from build123d import *

# Parameters (mm, degrees)
BOSS_EXTRUDE1_DEPTH = 3.175


with BuildPart() as part:
    # Sketch1 → Boss-Extrude1 (new body, symmetric)
    with BuildSketch(Plane(origin=(0, 0, 0), x_dir=(1, 0, 0), z_dir=(0, 1, 0))):
        Polygon((-203.2, 0), (203.2, 0), (203.2, 50.8), (82.55, 177.8), (-82.55, 177.8), (-203.2, 50.8), align=None)
    extrude(amount=BOSS_EXTRUDE1_DEPTH, both=True)


solid = part.part
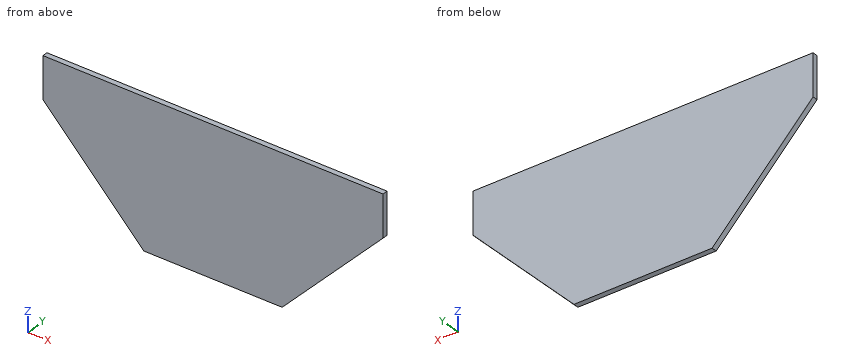
Geometry: final body of the model. Coordinates: model frame, mm. Give positions to 0.01 mm unless a question says otherwise; leave off trailing zeros. Loops run counter-clockwise (first coordinate to the right, second up) from the corner with the lowest first, then second, coordinate; pieces in that order, holes last. Notation, with made-up numbers: (-38.75, 46) - (-26.75, 46) arc R25 cw to (-26.75, 82) - close; hole circle Ø3 at (-26.75, 1). An arc over 180 degrees is marked (long way). One line per question, with ' | ' between items. Start each with the question number.
(1) Section query B-B on z = -72. Return loops of the section in (x, y) (3 decimals).
(2) Section query C-C on x = 121.5. Return loops of the section in (y, z) (3 decimals), then the cut area to 3 significant figures.
(3) Section query A-A on y = 1. Return loops of the section in (x, z).
(4) Ray query, line 1 (X direction, y = 1.5, z = -69.5) (3 decimals); line 2 (X direction, y = 0.5, z = -169.5) (3 decimals); line 3 (Z direction, x = -145.5, y = 2). Return the intervals inside material, ascending. Write a range as from..to.
The answers:
1) outline: (-183.06, -3.175) - (183.06, -3.175) - (183.06, 3.175) - (-183.06, 3.175) - close
2) outline: (-3.175, -136.8) - (3.175, -136.8) - (3.175, 0) - (-3.175, 0) - close | area: 869 mm2
3) outline: (-203.2, -50.8) - (-82.55, -177.8) - (82.55, -177.8) - (203.2, -50.8) - (203.2, 0) - (-203.2, 0) - close
4) line 1: -185.435..185.435 | line 2: -90.435..90.435 | line 3: -111.54..0
